For this review, take the finished solid that the model builds, in its own axes (mm). A direction names the side the tool comes from. Coordinates: 2 decimals unless noted, no trailing zeros. Write each loop counter-clockwise with the first axis right and the second up, starting at its lowest first coordinate (ties: lowest second). Pieces come first, ordered by that corner, then holes. Notation, with made-up numbers: M -12,1.5 L -1,1.5 A20 ccw -1,32.5 Z; hole C -38,85.25 d1. An arc over 180 degrees is marked long. One line per question, with ' | ' between items.
from build123d import *

# Parameters (mm, degrees)
SKETCH1_R           = 3
BOSS_EXTRUDE1_DEPTH = 2.5
SKETCH2_W           = 9
SKETCH2_H           = 4.761904762
BOSS_EXTRUDE2_DEPTH = 7.5
FILLET1_R           = 2
CHAMFER1_SIZE       = 1
FILLET2_R           = 1
SKETCH3_R           = 1.5
CUT_EXTRUDE1_DEPTH  = 20


with BuildPart() as part:
    # Sketch1 → Boss-Extrude1 (new body, symmetric)
    with BuildSketch(Plane.XY):
        with BuildLine():
            Line((0, 10), (-20, 10))
            Line((-20, 10), (-20, 0))
            Line((-20, 0), (-14, 0))
            Line((-14, 0), (-10, -4))
            Line((-10, -4), (-10, -10))
            Line((-10, -10), (0, -10))
            ThreePointArc((0, -10), (10, 0), (0, 10))
        make_face()
        Circle(SKETCH1_R, mode=Mode.SUBTRACT)
    extrude(amount=BOSS_EXTRUDE1_DEPTH, both=True)

    # Sketch2 → Boss-Extrude2 (add, symmetric)
    with BuildSketch(Plane.XY):
        with Locations((-15.5, 7.619047619)):
            Rectangle(SKETCH2_W, SKETCH2_H)
    extrude(amount=BOSS_EXTRUDE2_DEPTH, both=True)

    # Fillet1
    fillet1_edges = [part.edges().sort_by_distance(p)[0] for p in [
        (-15.5, 10, -7.5),
        (-15.5, 10, 7.5),
    ]]
    fillet(fillet1_edges, radius=FILLET1_R)

    # Chamfer1
    chamfer1_edges = [part.edges().sort_by_distance(p)[0] for p in [
        (-3, 0, -2.5),
        (-3, 0, 2.5),
    ]]
    chamfer(chamfer1_edges, length=CHAMFER1_SIZE)

    # Fillet2
    fillet2_edges = [part.edges().sort_by_distance(p)[0] for p in [
        (-5, -10, 2.5),
        (10, 0, 2.5),
        (-5.5, 10, 2.5),
        (-5.5, 10, -2.5),
        (10, 0, -2.5),
        (-5, -10, -2.5),
    ]]
    fillet(fillet2_edges, radius=FILLET2_R)

    # Sketch3 → Cut-Extrude1 (cut)
    with BuildSketch(Plane(origin=(0, 10, 0), x_dir=(1, 0, 0), z_dir=(0, 1, 0))):
        with Locations((-15, 0)):
            Circle(SKETCH3_R)
    extrude(amount=-CUT_EXTRUDE1_DEPTH, mode=Mode.SUBTRACT)


solid = part.part
1. Draft analysis for pull direction X (two halves, no side actions). For faces 5 (the cylindrical face through (-3, 0, 0)), 6 (the flat face through (-20, 6, 0)), 7 (the flat face through (-16, 7, 7.5)), state which applies: pulls with the +X half, pulls with the -X half, needs draft (parallel to the pull), parting line crosses it, or undercut.
Computed values:
face 5: undercut | face 6: pulls with the -X half | face 7: needs draft
2. Take a section at C-C on z = -3. State the section outline as (x, y) points, plus the area to 3 significant figures.
Computed values:
outline: M -20,5.24 L -11,5.24 L -11,10 L -20,10 Z | area: 42.9 mm2
3. Take a section at D-D on x = -13. State the section outline as (y, z) points.
Computed values:
outline: M -1,-2.5 L 5.24,-2.5 L 5.24,-7.5 L 8,-7.5 A2 ccw 10,-5.5 L 10,5.5 A2 ccw 8,7.5 L 5.24,7.5 L 5.24,2.5 L -1,2.5 Z
4. Clearance check with flat-ended pins moving along their axes: P1, Ø5, axis at y = -0.5, z = 4.5, coming from the +X side; P2, Ø5.5, axis at x = -8.5, y = 2.5, coming from the +Z side; P3, Ø4, axis at y = 8, z = 3.5, coming from the +X side. State where each tip first meets the part, or that it passes through.
Computed values:
P1: stops at x = 9.86 | P2: stops at z = 2.5 | P3: stops at x = 7.27
5. Take a section at B-B on y = 1.5. Give the number of separate pieces and of enclosed holes in the cut face, plus the area to 3 significant figures.
Computed values:
separate pieces: 2 | enclosed holes: 1 | area: 114 mm2
6. For line 1 along Z through (x, y) = (-15, 4); line 2 along Y through (x, z) = (0, -0.5); line 3 along Z through (x, y) = (-15, 6), list the stretches that pass through material, from the lowest coordinate up.
Computed values:
line 1: z = -2.5 to -1.5, 1.5 to 2.5 | line 2: y = -10 to -3, 3 to 10 | line 3: z = -7.5 to -1.5, 1.5 to 7.5
7. Machinability: for faces 1 (the cylindrical face through (-5.577, 9.715, 2.199)), 2 (the flat face through (-16, 5.238, -5)), 3 (the flat face through (-10, -7, 0)), 4 (the flat face through (-16, 5.238, 5)), which of the approach directions +Z, -Z, +X, -X, +Y, -Y give a long, thin tool a straight path to every point of the face, cutting with its end or side? Answer none if there is none.
Computed values:
face 1: +Z, +X, +Y | face 2: -Z, +X, -X, -Y | face 3: +Z, -Z, -X, -Y | face 4: +Z, +X, -X, -Y
8. Take a section at A-A on x = -9. State the section outline as (y, z) points.
Computed values:
outline: M -10,-1.5 A1 ccw -9,-2.5 L 9,-2.5 A1 ccw 10,-1.5 L 10,1.5 A1 ccw 9,2.5 L -9,2.5 A1 ccw -10,1.5 Z
